```python
from build123d import *

# Parameters (mm, degrees)
BOSS_EXTRUDE1_DEPTH = 3
SKETCH4_W           = 14
SKETCH4_H           = 3
CUT_EXTRUDE1_DEPTH  = 3
SKETCH5_R           = 1.5
CUT_EXTRUDE2_DEPTH  = 3
SKETCH6_W           = 11
SKETCH6_H           = 3.3
CUT_EXTRUDE3_DEPTH  = 3


with BuildPart() as part:
    # Sketch2 → Boss-Extrude1 (new body)
    with BuildSketch(Plane.XY):
        with BuildLine():
            Line((-1.603783622, 21.086206065), (-1.603783622, -2.133793935))
            ThreePointArc((-1.603783622, -2.133793935), (-2.189570059, -3.548007497), (-3.603783622, -4.133793935))
            Line((-3.603783622, -4.133793935), (-20.603783622, -4.133793935))
            ThreePointArc((-20.603783622, -4.133793935), (-22.017997184, -3.548007497), (-22.603783622, -2.133793935))
            Line((-22.603783622, -2.133793935), (-22.603783622, 16.166206065))
            ThreePointArc((-22.603783622, 16.166206065), (-22.017997184, 17.580419628), (-20.603783622, 18.166206065))
            Line((-20.603783622, 18.166206065), (-9.603783622, 18.166206065))
            ThreePointArc((-9.603783622, 18.166206065), (-8.896676841, 18.459099284), (-8.603783622, 19.166206065))
            Line((-8.603783622, 19.166206065), (-8.603783622, 21.086206065))
            ThreePointArc((-8.603783622, 21.086206065), (-5.103783622, 24.586206065), (-1.603783622, 21.086206065))
        make_face()
    extrude(amount=BOSS_EXTRUDE1_DEPTH)

    # Sketch4 → Cut-Extrude1 (cut)
    with BuildSketch(Plane.XY.offset(3)):
        with Locations((-10.603783622, 13.966206065)):
            Rectangle(SKETCH4_W, SKETCH4_H)
        with Locations((-15.603783622, 6.666206065)):
            Rectangle(SKETCH4_W, SKETCH4_H)
        with Locations((-15.603783622, 0.366206065)):
            Rectangle(SKETCH4_W, SKETCH4_H)
    extrude(amount=-CUT_EXTRUDE1_DEPTH, mode=Mode.SUBTRACT)

    # Sketch5 → Cut-Extrude2 (cut)
    with BuildSketch(Plane.XY.offset(3)):
        with Locations((-5.103783622, 21.086206065)):
            Circle(SKETCH5_R)
    extrude(amount=-CUT_EXTRUDE2_DEPTH, mode=Mode.SUBTRACT)

    # Sketch6 → Cut-Extrude3 (cut)
    with BuildSketch(Plane.XY.offset(3)):
        with Locations((-17.103783622, 3.516206065)):
            Rectangle(SKETCH6_W, SKETCH6_H)
    extrude(amount=-CUT_EXTRUDE3_DEPTH, mode=Mode.SUBTRACT)


solid = part.part
```
Design review of the part built by this model. Coordinates are the model's own, in mm. A direction names the side the tool comes from. Coordinates: 2 decimals unless noted, no trailing zeros. Write each loop counter-clockwise with the first axis right and the second up, starting at its lowest first coordinate (ties: lowest second). Pieces come first, ordered by that corner, then holes.
1) Add section B-B (z = 1.6). Write out the cut boundary in (x, y).
2) Add section A-A (y = 15). Write out the cut boundary in (x, z).
3) Add section C-C (x = -20). Write out the cut boundary in (y, z).
4) Mouldability with a two-part tool opening along X and no side actions: class faces 6 (the flat face through (-10, 5.166, 2)), 7 (the flat face through (-11, 15.466, 2)), 8 (the cylindrical face through (-8.904, 18.451, 1.479)), 9 (the cylindrical face through (-2.17, -3.53, 1.48)) as +X half, -X half, draft (parallel to the pull), parting line (faces both ways), or undercut.
5) Machinability: for faces 1 (the flat face through (-12, -4.134, 1)), 2 (the flat face through (-15, 18.166, 1)), 3 (the flat face through (-17.604, 14, 2)), 4 (the flat face through (-8.604, 7, 2)), 5 (the cylindrical face through (-22.002, -3.563, 1.479)), which of the approach directions +Z, -Z, +X, -X, +Y, -Y give a long, thin tool a straight path to every point of the face, cutting with its end or side? Answer none if there is none.
6) Add section D-D (x = -15). Write out the cut boundary in (y, z), plus the area to 3 significant figures.
7) Insertion check: pin 1 (0.6 mm diameter, centred on y = 20, z = 1, fed in from -X); pin 2 (1.5 mm diameter, centred on x = -10.5, z = 1.5, fed in from +Y); pin 3 (1.5 mm diameter, centred on y = 3, z = 1.5, fed in from -X). Each pin has a flat end and moves straight along its axis. Give the tip position at first contact, or say it passes through.
8) To check wall thickness, follow L1, parallel to Y at x = -5.25, z = 1.25; L2, parallel to Y at x = -9.75, z = 0.85; L3, parallel to Y at x = -19.75, z = 1.5. State the ranges of each line that lie inside material, in increasing order.
Check result:
1. outline: (-22.6, -2.13) arc R2 ccw to (-20.6, -4.13) - (-3.6, -4.13) arc R2 ccw to (-1.6, -2.13) - (-1.6, 21.09) arc R3.5 ccw to (-8.6, 21.09) - (-8.6, 19.17) arc R1 cw to (-9.6, 18.17) - (-20.6, 18.17) arc R2 ccw to (-22.6, 16.17) - (-22.6, 8.17) - (-8.6, 8.17) - (-8.6, 5.17) - (-11.6, 5.17) - (-11.6, 1.87) - (-8.6, 1.87) - (-8.6, -1.13) - (-22.6, -1.13) - close; hole (-17.6, 12.47) - (-3.6, 12.47) - (-3.6, 15.47) - (-17.6, 15.47) - close; hole circle Ø3 at (-5.1, 21.09)
2. outline: (-22.6, 0) - (-17.6, 0) - (-17.6, 3) - (-22.6, 3) - close; (-3.6, 0) - (-1.6, 0) - (-1.6, 3) - (-3.6, 3) - close
3. outline: (-4.13, 0) - (-1.13, 0) - (-1.13, 3) - (-4.13, 3) - close; (8.17, 0) - (18.17, 0) - (18.17, 3) - (8.17, 3) - close
4. face 6: draft
4. face 7: undercut
4. face 8: -X half
4. face 9: +X half
5. face 1: +Z, -Z, +X, -X, -Y
5. face 2: +Z, -Z, -X, +Y
5. face 3: +Z, -Z
5. face 4: +Z, -Z, -X
5. face 5: +Z, -Z, -X, -Y
6. outline: (-4.13, 0) - (-1.13, 0) - (-1.13, 3) - (-4.13, 3) - close; (8.17, 0) - (12.47, 0) - (12.47, 3) - (8.17, 3) - close; (15.47, 0) - (18.17, 0) - (18.17, 3) - (15.47, 3) - close
6. area: 30.0 mm2
7. pin 1: stops at x = -8.6
7. pin 2: stops at y = 18.17
7. pin 3: stops at x = -11.6
8. L1: y = -4.13 to 12.47, 15.47 to 19.59, 22.58 to 24.58
8. L2: y = -4.13 to -1.13, 1.87 to 5.17, 8.17 to 12.47, 15.47 to 18.17
8. L3: y = -4.13 to -1.13, 8.17 to 18.17
